Read the model definition and answer for the solid it produces. Units are mm, in the model's axes. A direction names the side the tool comes from. Round coordinates to 2 decimals unless told otherwise and drop trailing zeros. Write each loop counter-clockwise with the first axis right and the second up, starting at its lowest first coordinate (ties: lowest second). Pieces come first, ordered by that corner, then holes. Notation, with made-up numbers: (15.5, 19) -> (37.5, 19) arc R21 cw to (37.5, 30) -> close; hole circle Ø4 at (1, 24.5). An arc over 180 degrees is marked (long way). Return JSON: item names as keys, results as strings.
from build123d import *

# Parameters (mm, degrees)
F11_DEPTH = 5.59188
F6_R      = 1.3
F10_R     = 1.3
F9_R      = 1.3
F8_R      = 1.3
F7_R      = 1.3
F12_DEPTH = 12.5
F13_R     = 5
F14_R     = 7


with BuildPart() as f11:
    # F0 (on Front) → F11 (new body)
    with BuildSketch(Plane.XZ):
        with BuildLine():
            Line((-4.6259572574, 125.4466459383), (-18.9259572574, 125.4466459383))
            Line((-18.9259572574, 125.4466459383), (-18.9259572574, -30.7533540617))
            Line((-18.9259572574, -30.7533540617), (13.0740427426, -30.7533540617))
            Line((13.0740427426, -30.7533540617), (13.0740427426, -32.2533540617))
            Line((13.0740427426, -32.2533540617), (10.5740427426, -32.2533540617))
            Line((10.5740427426, -32.2533540617), (10.5740427426, -38.2533540617))
            Line((10.5740427426, -38.2533540617), (17.9395026739, -32.2533540617))
            Line((17.9395026739, -32.2533540617), (17.9395026739, -21.6533540617))
            Line((17.9395026739, -21.6533540617), (0.9395026739, -21.6533540617))
            ThreePointArc((0.9395026739, -21.6533540617), (2.3818043878, -11.7029252546), (-3.3089759276, -3.413999686))
            ThreePointArc((-3.3089759276, -3.413999686), (-5.7123935665, 3.262952785), (-3.3089759276, 9.939905256))
            ThreePointArc((-3.3089759276, 9.939905256), (3.3934420485, 20.2845633982), (-2.0037802352, 31.3662758301))
            ThreePointArc((-2.0037802352, 31.3662758301), (-3.7485817849, 35.5000324433), (-3.3089759276, 39.9653457441))
            ThreePointArc((-3.3089759276, 39.9653457441), (1.4696935081, 50.5333149606), (-4.6259572574, 60.4004673705))
            ThreePointArc((-4.6259572574, 60.4004673705), (-6.7621279189, 66.2099556499), (-4.6259572574, 72.0194439292))
            ThreePointArc((-4.6259572574, 72.0194439292), (1.9308894563, 81.7293683887), (-4.6259572574, 91.4392928481))
            ThreePointArc((-4.6259572574, 91.4392928481), (-7.770265303, 98.6246365011), (-4.6259572574, 105.809980154))
            ThreePointArc((-4.6259572574, 105.809980154), (0.9684001504, 115.6283130462), (-4.6259572574, 125.4466459383))
        make_face()
    extrude(amount=F11_DEPTH)

    # F6 (on line) + F10 (on line) + F9 (on line) + F8 (on line) + F7 (on line) → F12 (cut, symmetric)
    with BuildSketch(Plane(origin=(0, -2.2683734534, -0.5349668297), x_dir=(-1, 0, 0), z_dir=(0, 0.9732991931, 0.2295401504))):
        with Locations((4.6259572574, -9.8822513158)):
            Circle(F6_R)
    with BuildSketch(Plane(origin=(0, 25.6133496961, 6.0405805155), x_dir=(-1, 0, 0), z_dir=(0, 0.9732991931, 0.2295401504))):
        with Locations((4.6259572574, 111.5854879869)):
            Circle(F10_R)
    with BuildSketch(Plane(origin=(0, 18.6429189088, 4.3966936792), x_dir=(-1, 0, 0), z_dir=(0, 0.9732991931, 0.2295401504))):
        with Locations((4.6259572574, 81.2185531612)):
            Circle(F9_R)
    with BuildSketch(Plane(origin=(0, 11.6724881214, 2.7528068429), x_dir=(-1, 0, 0), z_dir=(0, 0.9732991931, 0.2295401504))):
        with Locations((4.6259572574, 50.8516183356)):
            Circle(F8_R)
    with BuildSketch(Plane(origin=(0, 4.702057334, 1.1089200066), x_dir=(-1, 0, 0), z_dir=(0, 0.9732991931, 0.2295401504))):
        with Locations((4.6259572574, 20.4846835099)):
            Circle(F7_R)
    extrude(amount=F12_DEPTH, both=True, mode=Mode.SUBTRACT)

    # F13
    f13_edges = [f11.edges().sort_by_distance(p)[0] for p in [
        (17.939503, -2.79594, -21.653354),
    ]]
    fillet(f13_edges, radius=F13_R)

    # F14
    f14_edges = [f11.edges().sort_by_distance(p)[0] for p in [
        (17.939503, -2.79594, -32.253354),
    ]]
    fillet(f14_edges, radius=F14_R)


solid = f11.part
Item 1: Section A-A (x = -12.5) is taken. Give the vertices of the cut face in (y, z), then the cut area to 3 significant figures.
Worked answers:
{"outline": "(-5.59, -30.75) -> (0, -30.75) -> (0, 125.45) -> (-5.59, 125.45) -> close", "area": "873 mm2"}
Item 2: Straight lines are drawn through the part: L1, parallel to Z at x = -15, y = -1.8; L2, parallel to X at y = -3.75, z = -15; L3, parallel to Z at x = 4, y = -1.65. For each, find the intervals that lie inside material, in ascending order. Write a range as [from, to].
Worked answers:
{"L1": "z = [-30.75, 125.45]", "L2": "x = [-18.93, 2.74]", "L3": "z = [-30.75, -21.65]"}
Item 3: For a pull along Z with two mould halves and no side action, classify faces 1 (the flat face through (12.934, -2.757, -36.331)), 2 (the flat face through (7, -3, -21.653)), 3 (the flat face through (-9, -5.592, 27)) as released by +Z, released by -Z, zero draft, split by the parting line, or undercut.
Worked answers:
{"face 1": "released by -Z", "face 2": "undercut", "face 3": "zero draft"}
Item 4: Section B-B (z = 29) is taken. Give the vertices of the cut face in (x, y), then the cut area to 3 significant figures.
Worked answers:
{"outline": "(-18.93, -5.59) -> (0.57, -5.59) -> (0.57, 0) -> (-18.93, 0) -> close", "area": "109 mm2"}
Item 5: A tool of negligible diameter and unlimited length cuts with its end or side. For faces 4 (the cylindrical face through (-5.827, -2.637, 19.913)), 5 (the flat face through (10.574, -3, -35)), from which of +Z, -Z, +X, -X, +Y, -Y can it reach the whole face along a straight path? Write none if from no direction.
Worked answers:
{"face 4": "none", "face 5": "-Z, -X, +Y, -Y"}
Item 6: Section C-C (y = -3.65) is taken. State how many separate pieces and enclosed holes the cut face has, then the cut area to 3 significant figures.
Worked answers:
{"separate pieces": "1", "enclosed holes": "5", "area": "2,900 mm2"}
Item 7: Flat-ended cylindrical pins translate along their axes: pin 1 (0.8 mm diameter, centred on x = 11.5, y = -2, fed in from +Z); pin 2 (8 mm diameter, centred on x = 3.5, z = 63.5, fed in from -Y); pin 3 (0.8 mm diameter, centred on y = -4, z = -31.5, fed in from -X). Find the tip coordinate at first contact, or state that the pin passes through.
Worked answers:
{"pin 1": "stops at z = -21.65", "pin 2": "passes through", "pin 3": "stops at x = 13.07"}
